from build123d import *

# Parameters (mm, degrees)
BOSS_EXTRUDE1_DEPTH   = 2
SKETCH2_R             = 2.35
BOSS_EXTRUDE2_DEPTH   = 4.5
BOSS_EXTRUDE3_START   = 6.5
BOSS_EXTRUDE3_DEPTH   = 2
BOSS_EXTRUDE4_START   = 29.415
SKETCH4_R             = 0.85
BOSS_EXTRUDE4_DEPTH   = 3
BOSS_EXTRUDE4_2_DEPTH = 3
BOSS_EXTRUDE4_3_DEPTH = 3
BOSS_EXTRUDE4_4_DEPTH = 3
SKETCH5_R             = 0.85
REVOLVE2_ANGLE        = 90
BOSS_EXTRUDE5_START   = -29.415
SKETCH4_2_R           = 0.85
BOSS_EXTRUDE5_DEPTH   = 3
BOSS_EXTRUDE5_2_DEPTH = 3
SKETCH6_R             = 0.85
REVOLVE3_ANGLE        = 90


with BuildPart() as part:
    # Sketch1 → Boss-Extrude1 (new body)
    with BuildSketch(Plane(origin=(0, 0, 0), x_dir=(1, 0, 0), z_dir=(0, 1, 0))):
        with BuildLine():
            ThreePointArc((-29.415, -15.875), (-28.734023266, -17.519023266), (-27.09, -18.2))
            Line((-27.09, -18.2), (27.09, -18.2))
            ThreePointArc((27.09, -18.2), (28.734023266, -17.519023266), (29.415, -15.875))
            Line((29.415, -15.875), (29.415, 15.875))
            ThreePointArc((29.415, 15.875), (28.734023266, 17.519023266), (27.09, 18.2))
            Line((27.09, 18.2), (-27.09, 18.2))
            ThreePointArc((-27.09, 18.2), (-28.734023266, 17.519023266), (-29.415, 15.875))
            Line((-29.415, 15.875), (-29.415, -15.875))
        make_face()
    extrude(amount=BOSS_EXTRUDE1_DEPTH)

    # Sketch2 → Boss-Extrude2 (add)
    with BuildSketch(Plane(origin=(0, 2, 0), x_dir=(1, 0, 0), z_dir=(0, 1, 0))):
        with Locations(Location((-27.09, -15.875, 0), (0, 0, 171.635124732))):
            Circle(SKETCH2_R)
        with Locations(Location((-27.09, 15.875, 0), (0, 0, 81.635124732))):
            Circle(SKETCH2_R)
        with Locations(Location((27.09, 15.875, 0), (0, 0, 98.364875268))):
            Circle(SKETCH2_R)
        with Locations(Location((27.09, -15.875, 0), (0, 0, 8.364875268))):
            Circle(SKETCH2_R)
    extrude(amount=BOSS_EXTRUDE2_DEPTH)

    # Sketch1<3> → Boss-Extrude3 (add)
    with BuildSketch(Plane(origin=(0, 0, 0), x_dir=(1, 0, 0), z_dir=(0, 1, 0)).offset(BOSS_EXTRUDE3_START)):
        with BuildLine():
            ThreePointArc((-29.415, -15.875), (-28.734023266, -17.519023266), (-27.09, -18.2))
            Line((-27.09, -18.2), (27.09, -18.2))
            ThreePointArc((27.09, -18.2), (28.734023266, -17.519023266), (29.415, -15.875))
            Line((29.415, -15.875), (29.415, 15.875))
            ThreePointArc((29.415, 15.875), (28.734023266, 17.519023266), (27.09, 18.2))
            Line((27.09, 18.2), (-27.09, 18.2))
            ThreePointArc((-27.09, 18.2), (-28.734023266, 17.519023266), (-29.415, 15.875))
            Line((-29.415, 15.875), (-29.415, -15.875))
        make_face()
    extrude(amount=BOSS_EXTRUDE3_DEPTH)



with BuildPart() as body_2:
    # Sketch4 → Boss-Extrude4 (new body)
    with BuildSketch(Plane(origin=(0, 0, 0), x_dir=(0, 0, -1), z_dir=(1, 0, 0)).offset(BOSS_EXTRUDE4_START)):
        with Locations((10.175, 2.85)):
            Circle(SKETCH4_R)
    extrude(amount=BOSS_EXTRUDE4_DEPTH)


with BuildPart() as body_3:
    # Sketch4 → Boss-Extrude4 2 (new body)
    with BuildSketch(Plane(origin=(0, 0, 0), x_dir=(0, 0, -1), z_dir=(1, 0, 0)).offset(BOSS_EXTRUDE4_START)):
        with Locations((6.175, 2.85)):
            Circle(SKETCH4_R)
    extrude(amount=BOSS_EXTRUDE4_2_DEPTH)


with BuildPart() as body_4:
    # Sketch4 → Boss-Extrude4 3 (new body)
    with BuildSketch(Plane(origin=(0, 0, 0), x_dir=(0, 0, -1), z_dir=(1, 0, 0)).offset(BOSS_EXTRUDE4_START)):
        with Locations((-6.175, 2.85)):
            Circle(SKETCH4_R)
    extrude(amount=BOSS_EXTRUDE4_3_DEPTH)


with BuildPart() as body_5:
    # Sketch4 → Boss-Extrude4 4 (new body)
    with BuildSketch(Plane(origin=(0, 0, 0), x_dir=(0, 0, -1), z_dir=(1, 0, 0)).offset(BOSS_EXTRUDE4_START)):
        with Locations((-10.175, 2.85)):
            Circle(SKETCH4_R)
    extrude(amount=BOSS_EXTRUDE4_4_DEPTH)


with BuildPart() as part_1:
    add(part.part)

    add(body_2.part)  # Revolve2 merges body 2

    add(body_3.part)  # Revolve2 merges body 3

    add(body_4.part)  # Revolve2 merges body 4

    add(body_5.part)  # Revolve2 merges body 5
    # Sketch5 → Revolve2 (revolve)
    with BuildSketch(Plane.ZY.offset(-29.415)):
        with Locations(Location((10.175, 2.85, 0), (0, 0, 270))):
            Circle(SKETCH5_R)
        with Locations(Location((6.175, 2.85, 0), (0, 0, 270))):
            Circle(SKETCH5_R)
        with Locations(Location((-6.175, 2.85, 0), (0, 0, 270))):
            Circle(SKETCH5_R)
        with Locations(Location((-10.175, 2.85, 0), (0, 0, 270))):
            Circle(SKETCH5_R)
    revolve(axis=Axis((29.415, 0, 0), (0, 0, 1)), revolution_arc=REVOLVE2_ANGLE)



with BuildPart() as body_2_2:
    # Sketch4<2> → Boss-Extrude5 (new body)
    with BuildSketch(Plane(origin=(0, 0, 0), x_dir=(0, 0, -1), z_dir=(1, 0, 0)).offset(BOSS_EXTRUDE5_START)):
        with Locations(Location((6.175, 2.85, 0), (0, 0, 270))):
            Circle(SKETCH4_2_R)
    extrude(amount=-BOSS_EXTRUDE5_DEPTH)


with BuildPart() as body_3_2:
    # Sketch4<2> → Boss-Extrude5 2 (new body)
    with BuildSketch(Plane(origin=(0, 0, 0), x_dir=(0, 0, -1), z_dir=(1, 0, 0)).offset(BOSS_EXTRUDE5_START)):
        with Locations(Location((10.175, 2.85, 0), (0, 0, 270))):
            Circle(SKETCH4_2_R)
    extrude(amount=-BOSS_EXTRUDE5_2_DEPTH)


with BuildPart() as part_2:
    add(part_1.part)

    add(body_2_2.part)  # Revolve3 merges body 2 2

    add(body_3_2.part)  # Revolve3 merges body 3 2
    # Sketch6 → Revolve3 (revolve)
    with BuildSketch(Plane(origin=(-29.415, 0, 0), x_dir=(0, 0, -1), z_dir=(1, 0, 0))):
        with Locations(Location((10.175, 2.85, 0), (0, 0, 270))):
            Circle(SKETCH6_R)
        with Locations(Location((6.175, 2.85, 0), (0, 0, 270))):
            Circle(SKETCH6_R)
    revolve(axis=Axis((-29.415, 0, 0), (0, 0, -1)), revolution_arc=REVOLVE3_ANGLE)


solid = part_2.part
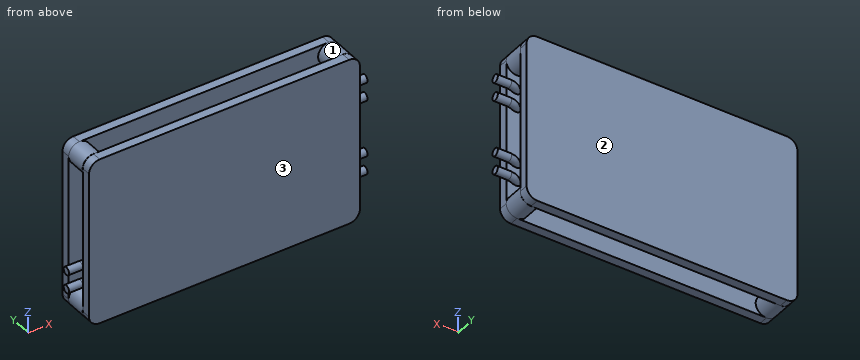
Could you check a few things on this model? Use its own coordinates, in mm. Face numbers are marked on the shaded views. Round coordinates to 2 decimals unless told otherwise and drop trailing zeros. Write each loop counter-clockwise with the first axis right and the second up, starting at its lowest first coordinate (ties: lowest second). Pieces come first, ordered by that corner, then holes. Notation, with made-up numbers: (-19, 43.5) - (35, 43.5) arc R16 ccw to (35, 62.5) - close; hole circle Ø5 at (73, 2). An arc over 180 degrees is marked (long way). Put each result on its own line as item: value. Start each with the question number.
(1) Thinking about a two-plate mould opening in Y: for the marked faces 1, 2 and 3, which applies, released by +Y, released by -Y, zero draft, split by the parting line, or undercut?
(2) I want a section at B-B, the plane x = 4. Please give me the cut outline in (y, z), plus the area to 3 significant figures.
(3) I want a section at C-C, the plane y = 2.85. Give the number of separate pieces and of enclosed holes in the cut face, plus the area to 3 significant figures.
(4) I need wall thicknesses on probe 1 along Y at (x, z) = (9.5, -4); probe 2 along X at (y, z) = (5.25, 16); probe 3 along Z at (x, y) = (28, 2.75). Which ranges of each line are inside material? Lowest first, please.
(5) I want a section at D-D, the plane y = 7.5. Please give me the cut outline in (x, z) (3 decimals), plus the area to 3 significant figures.
(6) Will these pins go through, and if not, where does the flat tip stop? pin 1 (0.6 mm diameter, centred on y = 1, z = -2.5, fed in from -X) (3 decimals); pin 2 (2 mm diameter, centred on x = 2, y = 7.5, fed in from -Z); pin 3 (4 mm diameter, centred on x = -6.5, y = 3.5, fed in from +Z).
(7) I want a section at A-A, the plane z = -1.5. Please give me the cut outline in (x, y) (3 decimals), plus the area to 3 significant figures.
Here are the results:
1. face 1: undercut
1. face 2: released by +Y
1. face 3: released by -Y
2. outline: (0, -18.2) - (2, -18.2) - (2, 18.2) - (0, 18.2) - close; (6.5, -18.2) - (8.5, -18.2) - (8.5, 18.2) - (6.5, 18.2) - close
2. area: 146 mm^2
3. separate pieces: 10
3. enclosed holes: 0
3. area: 121 mm^2
4. probe 1: y = 0 to 2, 6.5 to 8.5
4. probe 2: x = -29.44 to -24.74, 24.74 to 29.44
4. probe 3: z = -18.04 to -13.71, -10.99 to -9.36, -6.99 to -5.36, 5.36 to 6.99, 9.36 to 10.99, 13.71 to 18.04
5. outline: (-29.415, -15.875) arc R2.325 ccw to (-27.09, -18.2) - (27.09, -18.2) arc R2.325 ccw to (29.415, -15.875) - (29.415, 15.875) arc R2.325 ccw to (27.09, 18.2) - (-27.09, 18.2) arc R2.325 ccw to (-29.415, 15.875) - close
5. area: 2,140 mm^2
6. pin 1: stops at x = -29.415
6. pin 2: stops at z = -18.2
6. pin 3: stops at z = 18.2
7. outline: (-29.415, 0) - (29.415, 0) - (29.415, 2) - (-29.415, 2) - close; (-29.415, 6.5) - (29.415, 6.5) - (29.415, 8.5) - (-29.415, 8.5) - close
7. area: 235 mm^2
